Could you check a few things on this model? Use its own coordinates, in mm. Give positions to 0.01 mm unless a question says otherwise; leave off trailing zeros. Order: outer loops, then holes, each group sorted by start corner. A loop starts at its lowest first (then second) coordinate and runs counter-clockwise, first axis right, second up.
(1) Will these pins go through, and if not, where does the flat tip stop? pin 1 (12 mm diameter, centred on x = -41, y = 58, fed in from -Z); pin 2 (1.5 mm diameter, centred on x = 1, z = 1.5, fed in from -Y); pin 3 (2.5 mm diameter, centred on y = -84.5, z = 2.5, fed in from -X); pin 4 (2.5 mm diameter, centred on y = -85, z = 3, fed in from +X).
(2) Imagine slicing it at B-B, the plane x = 56. Write out the boundary of the cut face in (y, z), then the cut area to 3 significant figures.
(3) Imagine slicing it at A-A, the plane z = 3.15. State how many separate pieces and enclosed holes the cut face has, then the cut area to 3 significant figures.
(4) If I drill on probe 1 along Y at (x, z) = (140.5, 3.65); probe 2 along Y at (x, z) = (-59, 0.45); probe 3 along Y at (x, z) = (-19.5, 3.7), over which ranges is the centre line in solid material (lowest first)?
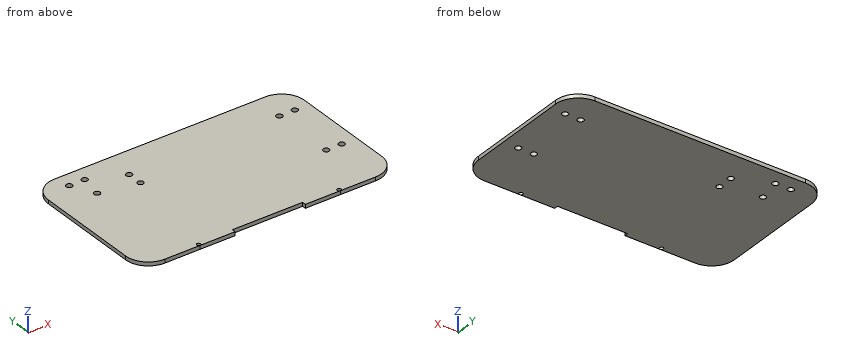
from build123d import *

# Parameters (mm, degrees)
CROQUIS1_R              = 4
SALIENTE_EXTRUIR1_DEPTH = 5
CROQUIS3_W              = 93.333333333
CROQUIS3_H              = 5
CORTAR_EXTRUIR1_DEPTH   = 10
CROQUIS6_R              = 2.5
CORTAR_EXTRUIR2_DEPTH   = 10


with BuildPart() as part:
    # Croquis1 → Saliente-Extruir1 (new body)
    with BuildSketch(Plane.XY):
        with BuildLine():
            Line((-125.472429705, -88.332065653), (154.527570295, -88.332065653))
            ThreePointArc((154.527570295, -88.332065653), (175.740773731, -79.545269088), (184.527570295, -58.332065653))
            Line((184.527570295, -58.332065653), (184.527570295, 81.667934347))
            ThreePointArc((184.527570295, 81.667934347), (175.740773731, 102.881137783), (154.527570295, 111.667934347))
            Line((154.527570295, 111.667934347), (-125.472429705, 111.667934347))
            ThreePointArc((-125.472429705, 111.667934347), (-146.68563314, 102.881137783), (-155.472429705, 81.667934347))
            Line((-155.472429705, 81.667934347), (-155.472429705, -58.332065653))
            ThreePointArc((-155.472429705, -58.332065653), (-146.68563314, -79.545269088), (-125.472429705, -88.332065653))
        make_face()
        with Locations((-105.472429705, 61.667934347)):
            Circle(CROQUIS1_R, mode=Mode.SUBTRACT)
        with Locations((-55.472429705, 71.667934347)):
            Circle(CROQUIS1_R, mode=Mode.SUBTRACT)
        with Locations((-55.472429705, 51.167934347)):
            Circle(CROQUIS1_R, mode=Mode.SUBTRACT)
        with Locations((144.027570295, -13.332065653)):
            Circle(CROQUIS1_R, mode=Mode.SUBTRACT)
        with Locations((164.527570295, -13.332065653)):
            Circle(CROQUIS1_R, mode=Mode.SUBTRACT)
        with Locations((144.027570295, 71.667934347)):
            Circle(CROQUIS1_R, mode=Mode.SUBTRACT)
        with Locations((164.527570295, 71.667934347)):
            Circle(CROQUIS1_R, mode=Mode.SUBTRACT)
        with Locations((-99.972429705, 91.667934347)):
            Circle(CROQUIS1_R, mode=Mode.SUBTRACT)
        with Locations((-120.472429705, 91.667934347)):
            Circle(CROQUIS1_R, mode=Mode.SUBTRACT)
    extrude(amount=SALIENTE_EXTRUIR1_DEPTH)

    # Croquis3 → Cortar-Extruir1 (cut)
    with BuildSketch(Plane.XY.offset(5)):
        with Locations((14.527570296, -85.832065653)):
            Rectangle(CROQUIS3_W, CROQUIS3_H)
    extrude(amount=-CORTAR_EXTRUIR1_DEPTH, mode=Mode.SUBTRACT)

    # Croquis6 → Cortar-Extruir2 (cut)
    with BuildSketch(Plane.XY.offset(5)):
        with Locations((-78.805763038, -85.842065653)):
            Circle(CROQUIS6_R)
        with Locations((107.860903629, -85.842065653)):
            Circle(CROQUIS6_R)
    extrude(amount=-CORTAR_EXTRUIR2_DEPTH, mode=Mode.SUBTRACT)


solid = part.part
Answer block:
1. pin 1: stops at z = 0
1. pin 2: stops at y = -83.33
1. pin 3: stops at x = -142.18
1. pin 4: stops at x = 170.46
2. outline: (-83.33, 0) - (111.67, 0) - (111.67, 5) - (-83.33, 5) - close
2. area: 975 mm2
3. separate pieces: 1
3. enclosed holes: 9
3. area: 66,300 mm2
4. probe 1: y = -88.33 to -15.22, -11.45 to 69.78, 73.55 to 111.67
4. probe 2: y = -88.33 to 49.28, 53.05 to 69.78, 73.55 to 111.67
4. probe 3: y = -83.33 to 111.67
